from build123d import *

# Parameters (mm, degrees)
EXTRUDE1_DEPTH             = 12.7
ARC_MOUNTING_SLOT_I_DEPTH  = 48.184559381
CLAMPING_SCREW_HOLES_D     = 5.1054
CLAMPING_SCREW_HOLES_DEPTH = 15.24
CLAMPING_SCREW_HOLES_TIP   = 1.533816902


with BuildPart() as part:
    # Sketch1 → Extrude1 (new, symmetric)
    with BuildSketch(Plane.XY):
        Polygon((-12.7, 44.8056), (10.16, 44.8056), (10.16, 29.5656), (0, 29.5656), (0, 12.2936), (12.7, 12.2936), (31.75, 12.2936), (31.75, 0), (-31.75, 0), (-31.75, 12.2936), (-12.7, 12.2936), align=None)
    extrude(amount=EXTRUDE1_DEPTH, both=True)

    # Sketch2 → Arc mounting slot I (cut, through all)
    with BuildSketch(Plane(origin=(0, 12.2936, 0), x_dir=(-1, 0, 0), z_dir=(0, 1, 0))):
        with BuildLine():
            ThreePointArc((-25.839582785, -4.556215615), (-21.92608696, -7.296474893), (-19.185827683, -3.382979068))
            ThreePointArc((-19.185827683, -3.382979068), (-19.4818, 0), (-19.185827683, 3.382979068))
            ThreePointArc((-19.185827683, 3.382979068), (-21.92608696, 7.296474893), (-25.839582785, 4.556215615))
            ThreePointArc((-25.839582785, 4.556215615), (-26.2382, 0), (-25.839582785, -4.556215615))
        make_face()
    arc_mounting_slot_i = extrude(amount=-ARC_MOUNTING_SLOT_I_DEPTH, mode=Mode.SUBTRACT)

    # Arc mounting slot II: Arc mounting slot I across plane
    add(arc_mounting_slot_i.mirror(Plane(origin=(0, 0, 0), x_dir=(0, 0, 1), z_dir=(1, 0, 0))), mode=Mode.SUBTRACT)

    # Clamping screw holes
    with Locations(Plane(origin=(0, 44.8056, 0), x_dir=(-1, 0, 0), z_dir=(0, 1, 0))):
        with Locations((-3.96875, -7.9375), (-3.96875, 7.9375)):
            Hole(CLAMPING_SCREW_HOLES_D / 2, depth=CLAMPING_SCREW_HOLES_DEPTH)
            with Locations((0, 0, -(CLAMPING_SCREW_HOLES_DEPTH + CLAMPING_SCREW_HOLES_TIP / 2))):  # 118° drill point
                Cone(0, CLAMPING_SCREW_HOLES_D / 2, CLAMPING_SCREW_HOLES_TIP, mode=Mode.SUBTRACT)


solid = part.part
Build history of the part. All positions in model axes, mm. A direction names the side the tool comes from. Round coordinates to 2 decimals unless told otherwise and drop trailing zeros. Write each loop counter-clockwise with the first axis right and the second up, starting at its lowest first coordinate (ties: lowest second). Pieces come first, ordered by that corner, then holes. Notation, with made-up numbers: (-26.5, 80.25) - (8.5, 80.25) arc R21 cw to (8.5, 94.25) - close; hole circle Ø7 at (-33.5, 58). An arc over 180 degrees is marked (long way). One line per question, with ' | ' between items.
1. Drop flat-ended pins along their axis: pin 1 Ø12 at (y, z) = (30.5, -3) entering from +X; pin 2 Ø1.5 at (x, z) = (24.5, 0.5) entering from -Y; pin 3 Ø1 at (y, z) = (13, -5.5) entering from -X; pin 4 Ø5.5 at (x, z) = (-21.5, -6.5) entering from +Y. Give the stop position or say it passes through.
Results are:
pin 1: x = 10.16 | pin 2: through | pin 3: x = -12.7 | pin 4: y = 12.29
2. Band-saw the part on D-D, the plane z = -6.25. Write the cut outline in (x, y).
Results are:
outline: (-31.75, 0) - (-25.01, 0) - (-25.01, 12.29) - (-31.75, 12.29) - close; (-20.02, 0) - (20.02, 0) - (20.02, 12.29) - (0, 12.29) - (0, 29.57) - (2.05, 29.57) - (2.05, 44.81) - (-12.7, 44.81) - (-12.7, 12.29) - (-20.02, 12.29) - close; (5.88, 29.57) - (10.16, 29.57) - (10.16, 44.81) - (5.88, 44.81) - close; (25.01, 0) - (31.75, 0) - (31.75, 12.29) - (25.01, 12.29) - close
3. Band-saw the part on B-B, the plane x = 5. Write the cut outline in (y, z).
Results are:
outline: (0, -12.7) - (12.29, -12.7) - (12.29, 12.7) - (0, 12.7) - close; (29.57, -12.7) - (44.81, -12.7) - (44.81, -10.27) - (29.57, -10.27) - close; (29.57, -5.6) - (44.81, -5.6) - (44.81, 5.6) - (29.57, 5.6) - close; (29.57, 10.27) - (44.81, 10.27) - (44.81, 12.7) - (29.57, 12.7) - close
4. Tool access for faces 1 (the face through (19.48, 6.23, -0.05)), 2 (the face through (-7, 18, 12.7)), 3 (the face through (-12.7, 28, 0)), 4 (the face through (10.16, 37, 0)), 5 (the face through (3.42, 37.08, -10.43)): list every direction of +Z, -Z, +X, -X, +Y, -Y with a clear straight run to the whole face (end or side of a thin tool).
Results are:
face 1: +Y, -Y | face 2: +Z, +X, -X, +Y, -Y | face 3: +Z, -Z, -X, +Y | face 4: +Z, -Z, +X, +Y | face 5: +Y
5. Drill centre lines: line 1 along Y through (x, z) = (9.5, 6.5); line 2 along Y through (x, z) = (15.5, -8.5); line 3 along X through (y, z) = (16, 9.25). Where is each one in solid material? Low to high. Write a range as from..to.
Results are:
line 1: 0..12.29, 29.57..44.81 | line 2: 0..12.29 | line 3: -12.7..0
6. Mould opens along Y. For faces 6 (the face through (0, 21, 0)), 7 (the face through (5, 29.566, 0)), 8 (the face through (22, 6.23, -7.31)), 9 (the face through (-18, 12.294, 0)) say: released by +Y, released by -Y, zero draft, split by the parting line, or undercut.
Results are:
face 6: undercut | face 7: undercut | face 8: zero draft | face 9: released by +Y
7. Band-saw the part on C-C, the plane y = 3. Write the cut outline in (x, z).
Results are:
outline: (-31.75, -12.7) - (31.75, -12.7) - (31.75, 12.7) - (-31.75, 12.7) - close; hole (-25.84, -4.56) arc R3.38 ccw to (-19.19, -3.38) arc R19.48 cw to (-19.19, 3.38) arc R3.38 ccw to (-25.84, 4.56) arc R26.24 ccw to start; hole (19.19, -3.38) arc R3.38 ccw to (25.84, -4.56) arc R26.24 ccw to (25.84, 4.56) arc R3.38 ccw to (19.19, 3.38) arc R19.48 cw to start
8. Band-saw the part on A-A, the plane z = -2.5. Write the cut outline in (x, y).
Results are:
outline: (-31.75, 0) - (-26.12, 0) - (-26.12, 12.29) - (-31.75, 12.29) - close; (-19.32, 0) - (19.32, 0) - (19.32, 12.29) - (0, 12.29) - (0, 29.57) - (10.16, 29.57) - (10.16, 44.81) - (-12.7, 44.81) - (-12.7, 12.29) - (-19.32, 12.29) - close; (26.12, 0) - (31.75, 0) - (31.75, 12.29) - (26.12, 12.29) - close
